```python
from build123d import *

# Parameters (mm, degrees)
SKETCH_2_R      = 1.6
EXTRUDE_1_DEPTH = 4


with BuildPart() as part:
    # 草图2 → 凸台-拉伸1 (new body)
    with BuildSketch(Plane(origin=(0, 0, 0), x_dir=(1, 0, 0), z_dir=(0, 1, 0))):
        with BuildLine():
            Line((-21.264895519, 46.809256481), (4.693469915, 46.809256481))
            ThreePointArc((4.693469915, 46.809256481), (-20.764895519, 1.809256481), (4.693469915, -43.190743519))
            Line((4.693469915, -43.190743519), (-21.264895519, -43.190743519))
            Line((-21.264895519, -43.190743519), (-21.264895519, -14.190743519))
            Line((-21.264895519, -14.190743519), (-26.264895519, -4.190743519))
            Line((-26.264895519, -4.190743519), (-41.264895519, -4.190743519))
            Line((-41.264895519, -4.190743519), (-41.264895519, 7.809256481))
            Line((-41.264895519, 7.809256481), (-26.264895519, 7.809256481))
            Line((-26.264895519, 7.809256481), (-21.264895519, 17.809256481))
            Line((-21.264895519, 17.809256481), (-21.264895519, 46.809256481))
        make_face()
        with Locations((-36.264895519, 1.809256481)):
            Circle(SKETCH_2_R, mode=Mode.SUBTRACT)
        with Locations((-26.264895519, 1.809256481)):
            Circle(SKETCH_2_R, mode=Mode.SUBTRACT)
    extrude(amount=EXTRUDE_1_DEPTH)


solid = part.part
```
For this review, take the finished solid that the model builds, in its own axes (mm). A direction names the side the tool comes from. Coordinates: 2 decimals unless noted, no trailing zeros. Loops run counter-clockwise (first coordinate to the right, second up) from the corner with the lowest first, then second, coordinate; pieces in that order, holes last. Notation, with made-up numbers: (-12.5, 1.5) -> (32.5, 1.5) arc R19 cw to (32.5, 19.5) -> close; hole circle Ø2 at (-11.75, 34.5). An arc over 180 degrees is marked (long way). Return JSON: item names as keys, results as strings. Group by question number.
(1) Consider section D-D, the plane z = 26. Give the boundary of the cut face in (x, y).
(2) Tool access review of faces 1 (the flat face through (-34, 2, 4.191)), 2 (the flat face through (-8, 2, -46.809)), 3 (the flat face through (-34, 2, -7.809)): name each direction out of +Z, -Z, +X, -X, +Y, -Y from which nothing blocks a thin tool from reaching the whole face with its end or side.
(3) For pin 1 Ø8 at (x, z) = (-15.5, -9.5) entering from -Y; pin 2 Ø1.2 at (y, z) = (3, 26) entering from -X, all flat-tipped, find the tip position at first contact; note any pin that passes through.
(4) Mouldability with a two-part tool opening along X and no side actions: class faces 4 (the flat face through (-8, 2, 43.191)), 5 (the cylindrical face through (-34.74, 1.97, -2.29)), 6 (the flat face through (-23.73, 1.97, 9.26)), 7 (the cylindrical face through (-20.76, 1.97, -2.57)) as pulls with the +X half, pulls with the -X half, needs draft (parallel to the pull), parting line crosses it, or undercut.
(5) Consider section C-C, the plane x = -8.5. Give the boundary of the cut face in (y, z).
(6) Consider section A-A, the plane x = -17.5. Give the boundary of the cut face in (y, z).
(7) To check wall thickness, follow L1, parallel to Z at x = -33, y = 3.45; L2, parallel to Z at x = -35.5, y = 2; L3, parallel to Z at x = -6, y = 2.5. State the ranges of each line that lie inside material, in increasing order.
(8) Consider section B-B, the plane y = 2.35. Give the boundary of the cut face in (x, z), plus the area to 3 significant figures.
Results below:
{
 "1": {"outline": "(-21.26, 0) -> (-12.79, 0) -> (-12.79, 4) -> (-21.26, 4) -> close"},
 "2": {"face 1": "+Z, -X, +Y, -Y", "face 2": "-Z, +X, -X, +Y, -Y", "face 3": "-Z, -X, +Y, -Y"},
 "3": {"pin 1": "passes through", "pin 2": "stops at x = -21.26"},
 "4": {"face 4": "needs draft", "face 5": "undercut", "face 6": "pulls with the -X half", "face 7": "pulls with the +X half"},
 "5": {"outline": "(0, -46.81) -> (4, -46.81) -> (4, -35.53) -> (0, -35.53) -> close; (0, 31.92) -> (4, 31.92) -> (4, 43.19) -> (0, 43.19) -> close"},
 "6": {"outline": "(0, -46.81) -> (4, -46.81) -> (4, -20.03) -> (0, -20.03) -> close; (0, 16.42) -> (4, 16.42) -> (4, 43.19) -> (0, 43.19) -> close"},
 "7": {"L1": "z = -7.81 to 4.19", "L2": "z = -7.81 to -3.21, -0.4 to 4.19", "L3": "z = -46.81 to -38.31, 34.69 to 43.19"},
 "8": {"outline": "(-41.26, -7.81) -> (-26.26, -7.81) -> (-21.26, -17.81) -> (-21.26, -46.81) -> (4.69, -46.81) arc R52.5 cw to (4.69, 43.19) -> (-21.26, 43.19) -> (-21.26, 14.19) -> (-26.26, 4.19) -> (-41.26, 4.19) -> close; hole circle Ø3.2 at (-36.26, -1.81); hole circle Ø3.2 at (-26.26, -1.81)", "area": "989 mm2"}
}
